Work out the finished part from the listing and answer in its coordinate system (mm). Face numbers are marked on the shaded views. A direction names the side the tool comes from. Give positions to 0.01 mm unless a question says otherwise; leave off trailing zeros. Order: outer loops, then holes, each group sorted by start corner. A loop starts at its lowest first (then second) coordinate and runs counter-clockwise, first axis right, second up. Notation, with made-up numbers: (46, -22.75) -> (92, -22.75) arc R25 cw to (92, 9.25) -> close; hole circle Ø11 at (4, 81). An arc over 180 degrees is marked (long way). Answer as CSV lines item,"result". Start each with the question number.
1. For a pull along Z with two mould halves and no side action, classify the marked faces 1, 2, 3 and 4 as released by +Z, released by -Z, zero draft, split by the parting line, or undercut.
2. A cutting plane is placed at C-C (z = 51.5). Give the vertices of the cut face in (x, y).
3. Find the intervals of material crossed by L1, parallel to Y at x = 72, z = 0; L2, parallel to Y at x = 99, z = 0; L3, parallel to Y at x = 112.5, z = 16.5, in increasing order.
4. Flat-ended cylindrical pins translate along their axes: pin 1 (12 mm diameter, centred on y = -48.5, z = -26.5, fed in from -X); pin 2 (3 mm diameter, centred on x = 95, z = 33, fed in from +Y); pin 3 (0.9 mm diameter, centred on x = 66.5, y = -16, fed in from +Z). Find the tip coordinate at first contact, or state that the pin passes through.
5. A cutting plane is placed at A-A (z = -29). Give the vertices of the cut face in (x, y), then the cut area to 3 significant figures.
6. A cutting plane is placed at B-B (y = -49.5). Give the vertices of the cut face in (x, z).
7. For the marked faces 5, 6 and 7, determine the directions among +Z, -Z, +X, -X, +Y, -Y from which every point of the face is accessible in a straight line to the end or side of a thin tool.
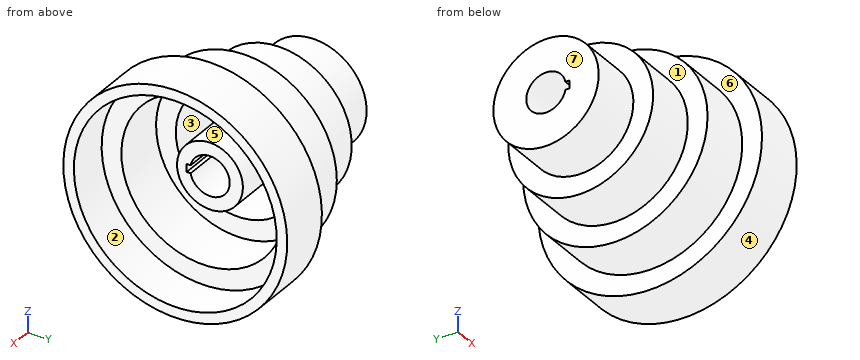
from build123d import *

# Parameters (mm, degrees)
CUT_EXTRUDE1_DEPTH      = 201.124960962
CUT_EXTRUDE1_DEPTH_BACK = 201.124960962


with BuildPart() as part:
    # Sketch2 → Revolve1 (revolve)
    with BuildSketch(Plane.XY, mode=Mode.PRIVATE) as revolve1_sk:
        Polygon((0, 15), (120, 15), (120, 25), (48, 25), (48, 47), (88, 47), (88, 62), (128, 62), (128, 77), (160, 77), (160, 85), (120, 85), (120, 70), (80, 70), (80, 55), (40, 55), (40, 40), (0, 40), align=None)
    revolve(revolve1_sk.sketch.rotate(Axis((-111.650485437, 0, 0), (1, 0, 0)), 90), axis=Axis((-111.650485437, 0, 0), (1, 0, 0)))

    # Sketch3 → Cut-Extrude1 (cut, two sides: drawn at the far end of the back side and taken through both)
    with BuildSketch(Plane.ZY.offset(-CUT_EXTRUDE1_DEPTH_BACK)):
        with BuildLine():
            Line((-3, -14.696938457), (-3, -17.696938457))
            Line((-3, -17.696938457), (3, -17.696938457))
            Line((3, -17.696938457), (3, -14.696938457))
            ThreePointArc((3, -14.696938457), (0, 15), (-3, -14.696938457))
        make_face()
    extrude(amount=CUT_EXTRUDE1_DEPTH + CUT_EXTRUDE1_DEPTH_BACK, mode=Mode.SUBTRACT)


solid = part.part
Answer sheet:
1,face 1,"zero draft"
1,face 2,"undercut"
1,face 3,"undercut"
1,face 4,"split by the parting line"
2,outline,"(40, -19.31) -> (80, -19.31) -> (80, -47.41) -> (120, -47.41) -> (120, -67.62) -> (160, -67.62) -> (160, -57.24) -> (128, -57.24) -> (128, -34.52) -> (88, -34.52) -> (88, 34.52) -> (128, 34.52) -> (128, 57.24) -> (160, 57.24) -> (160, 67.62) -> (120, 67.62) -> (120, 47.41) -> (80, 47.41) -> (80, 19.31) -> (40, 19.31) -> close"
3,L1,"y = -55 to -47, -25 to -17.7, 15 to 25, 47 to 55"
3,L2,"y = -70 to -62, -25 to -17.7, 15 to 25, 62 to 70"
3,L3,"y = -68.03 to -59.76, -18.78 to 18.78, 59.76 to 68.03"
4,pin 1,"stops at x = 40"
4,pin 2,"stops at y = 62.51"
4,pin 3,"stops at z = 52.76"
5,outline,"(0, -27.55) -> (40, -27.55) -> (40, -46.73) -> (80, -46.73) -> (80, -63.71) -> (120, -63.71) -> (120, -79.9) -> (160, -79.9) -> (160, -71.33) -> (128, -71.33) -> (128, -54.8) -> (88, -54.8) -> (88, -36.99) -> (48, -36.99) -> (48, 36.99) -> (88, 36.99) -> (88, 54.8) -> (128, 54.8) -> (128, 71.33) -> (160, 71.33) -> (160, 79.9) -> (120, 79.9) -> (120, 63.71) -> (80, 63.71) -> (80, 46.73) -> (40, 46.73) -> (40, 27.55) -> (0, 27.55) -> close"
5,area,"5,520 mm^2"
6,outline,"(40, -23.97) -> (80, -23.97) -> (80, -49.49) -> (120, -49.49) -> (120, -69.1) -> (160, -69.1) -> (160, -58.98) -> (128, -58.98) -> (128, -37.33) -> (88, -37.33) -> (88, 37.33) -> (128, 37.33) -> (128, 58.98) -> (160, 58.98) -> (160, 69.1) -> (120, 69.1) -> (120, 49.49) -> (80, 49.49) -> (80, 23.97) -> (40, 23.97) -> close"
7,face 5,"+X"
7,face 6,"-X"
7,face 7,"+Z, -Z, -X, +Y, -Y"
